Source: CAD feature listing. Evaluate the final solid. Frame: model axes, mm. Face numbers are marked on the shaded views. A direction names the side the tool comes from. Give positions to 0.01 mm unless a question says otherwise; leave off trailing zeros. Write each loop counter-clockwise with the first axis right and the second up, starting at its lowest first coordinate (ties: lowest second). Pieces come first, ordered by that corner, then holes. Notation, with made-up numbers: (-40, 63.5) -> (7, 63.5) arc R20 cw to (7, 95.5) -> close; hole circle Ø11 at (-0.75, 10.5). An arc over 180 degrees is marked (long way). Answer as a JSON object with one key per item and string values. Group by question number.
Item 1: Section query D-D on y = -0.5. Return the cut outline in (x, z), plus the area to 3 significant figures.
Item 2: First-contact query: pin 1 Ø2.5 at (x, y) = (18.5, -0.5) entering from -Z. Flat tip, straight axial feed; report the tip coordinate or a pass-through.
Item 3: Section query C-C on x = 26. Return the cut outline in (y, z), plus the area to 3 significant figures.
Item 4: Section query A-A on y = -2.25. Return the cut outline in (x, z), plus the area to 3 significant figures.
Item 5: Section query B-B on z = 2.1. Return the cut outline in (x, y).
Item 6: Access query for the marked faces 5 and 6. Directions: +Z, -Z, +X, -X, +Y, -Y. A direction counts if a zero-diameter tool reaches every point of the face in a straight line with its end or side. Return the directions, or none.
Item 7: Ray query, probe 1 along Y at (x, z) = (0, 2.75); probe 2 along X at (y, z) = (-0.75, 1.35); probe 3 along Y at (x, z) = (-1, 1.6). Return the intervals inside material, ascending. Write a range as from..to.
Item 8: Pull-direction query (Y, two-part tool) for the marked faces 1, 2, 3 and 4; classes: pulls with the +Y half, pulls with the -Y half, needs draft (parallel to the pull), parting line crosses it, or undercut.
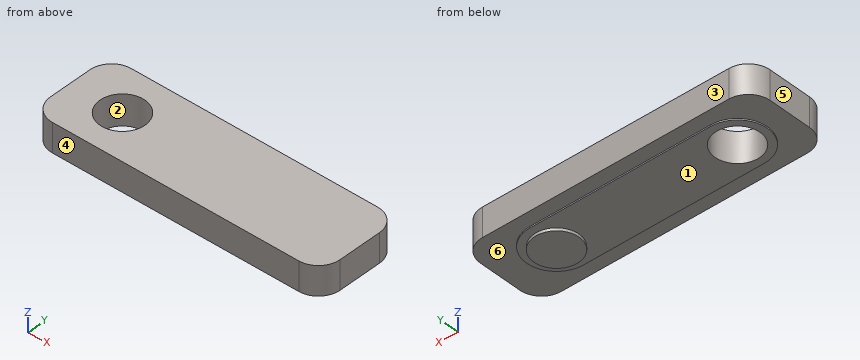
from build123d import *

# Parameters (mm, degrees)
F2_DEPTH = 0.2
F0_W     = 40
F0_H     = 12
F4_DEPTH = 4
F5_R     = 3
F7_D     = 6.2
F3_R     = 3.1
F8_DEPTH = 0.6


with BuildPart() as f2:
    # F1 (on Top) → F2 (new body)
    with BuildSketch(Plane.XY):
        with BuildLine():
            ThreePointArc((0, -4.1), (2.899138, -2.899138), (4.1, 0))
            ThreePointArc((4.1, 0), (2.899138, 2.899138), (0, 4.1))
            ThreePointArc((0, 4.1), (-4.1, 0), (0, -4.1))
        make_face()
        with BuildLine():
            ThreePointArc((0, 4.1), (2.899138, 2.899138), (4.1, 0))
            ThreePointArc((4.1, 0), (2.899138, -2.899138), (0, -4.1))
            Line((0, -4.1), (25, -4.1))
            ThreePointArc((25, -4.1), (20.9, 0), (25, 4.1))
            Line((25, 4.1), (0, 4.1))
        make_face()
        with BuildLine():
            ThreePointArc((29.1, 0), (27.899138, 2.899138), (25, 4.1))
            ThreePointArc((25, 4.1), (20.9, 0), (25, -4.1))
            ThreePointArc((25, -4.1), (27.899138, -2.899138), (29.1, 0))
        make_face()
    extrude(amount=-F2_DEPTH)

    # F0 (on Top) → F4 (join)
    with BuildSketch(Plane.XY):
        with Locations((12.779413, 0)):
            Rectangle(F0_W, F0_H)
    extrude(amount=F4_DEPTH)

    # F5
    f5_edges = [f2.edges().sort_by_distance(p)[0] for p in [
        (32.779413, -6, 2),
        (32.779413, 6, 2),
        (-7.220587, -6, 2),
        (-7.220587, 6, 2),
    ]]
    fillet(f5_edges, radius=F5_R)

    # F7 (through all)
    with Locations(Plane.XY.offset(4)):
        with Locations((0, 0)):
            Hole(F7_D / 2)

    # F3 (on Top) → F8 (join)
    with BuildSketch(Plane.XY):
        with Locations((25, 0)):
            Circle(F3_R)
    extrude(amount=-F8_DEPTH)


solid = f2.part
Worked answers:
{
 "1": {"outline": "(-7.22, 0) -> (-4.07, 0) -> (-4.07, -0.2) -> (-3.06, -0.2) -> (-3.06, 4) -> (-7.22, 4) -> close; (3.06, -0.2) -> (21.94, -0.2) -> (21.94, -0.6) -> (28.06, -0.6) -> (28.06, -0.2) -> (29.07, -0.2) -> (29.07, 0) -> (32.78, 0) -> (32.78, 4) -> (3.06, 4) -> close", "area": "143 mm^2"},
 "2": {"pin 1": "z = -0.2"},
 "3": {"outline": "(-6, 0) -> (-3.98, 0) -> (-3.98, -0.2) -> (-2.93, -0.2) -> (-2.93, -0.6) -> (2.93, -0.6) -> (2.93, -0.2) -> (3.98, -0.2) -> (3.98, 0) -> (6, 0) -> (6, 4) -> (-6, 4) -> close", "area": "51.9 mm^2"},
 "4": {"outline": "(-7.22, 0) -> (-3.43, 0) -> (-3.43, -0.2) -> (-2.13, -0.2) -> (-2.13, 4) -> (-7.22, 4) -> close; (2.13, -0.2) -> (22.87, -0.2) -> (22.87, -0.6) -> (27.13, -0.6) -> (27.13, -0.2) -> (28.43, -0.2) -> (28.43, 0) -> (32.78, 0) -> (32.78, 4) -> (2.13, 4) -> close", "area": "150 mm^2"},
 "5": {"outline": "(-7.22, -3) arc R3 ccw to (-4.22, -6) -> (29.78, -6) arc R3 ccw to (32.78, -3) -> (32.78, 3) arc R3 ccw to (29.78, 6) -> (-4.22, 6) arc R3 ccw to (-7.22, 3) -> close; hole circle Ø6.2 at (0, 0)"},
 "6": {"face 5": "+Z, -Z, -X, +Y, -Y", "face 6": "-Z"},
 "7": {"probe 1": "-6..-3.1, 3.1..6", "probe 2": "-7.22..-3.01, 3.01..32.78", "probe 3": "-6..-2.93, 2.93..6"},
 "8": {"face 1": "needs draft", "face 2": "undercut", "face 3": "pulls with the +Y half", "face 4": "pulls with the -Y half"}
}
